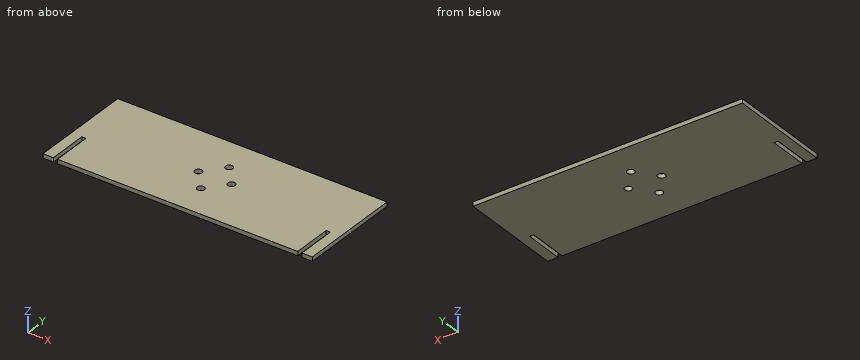
from build123d import *

# Parameters (mm, degrees)
SKETCH1_R           = 1.75
BOSS_EXTRUDE1_DEPTH = 1


with BuildPart() as part:
    # Sketch1 → Boss-Extrude1 (new, symmetric)
    with BuildSketch(Plane.XY):
        Polygon((-65, 25), (65, 25), (65, -25), (60, -25), (60, -6), (58, -6), (58, -25), (-58, -25), (-58, -6), (-60, -6), (-60, -25), (-65, -25), align=None)
        with Locations((0, 9.5)):
            Circle(SKETCH1_R, mode=Mode.SUBTRACT)
        with Locations((8, 0)):
            Circle(SKETCH1_R, mode=Mode.SUBTRACT)
        with Locations((0, -9.5)):
            Circle(SKETCH1_R, mode=Mode.SUBTRACT)
        with Locations((-8, 0)):
            Circle(SKETCH1_R, mode=Mode.SUBTRACT)
    extrude(amount=BOSS_EXTRUDE1_DEPTH, both=True)


solid = part.part
CAD build for the part. Positions are in the model's coordinates, mm. Give positions to 0.01 mm unless a question says otherwise; leave off trailing zeros. Write each loop counter-clockwise with the first axis right and the second up, starting at its lowest first coordinate (ties: lowest second). Pieces come first, ordered by that corner, then holes. Notation, with made-up numbers: (59, 17.5) -> (100, 17.5) arc R13 ccw to (100, 34.5) -> close; hole circle Ø3 at (54, 36). An arc over 180 degrees is marked (long way). Return JSON: item names as keys, results as strings.
Item 1: Band-saw the part on A-A (y = -20). List the corners of the cut face in (x, z), then the cut area to 3 significant figures.
Answer below:
{"outline": "(-65, -1) -> (-60, -1) -> (-60, 1) -> (-65, 1) -> close; (-58, -1) -> (58, -1) -> (58, 1) -> (-58, 1) -> close; (60, -1) -> (65, -1) -> (65, 1) -> (60, 1) -> close", "area": "252 mm2"}
Item 2: Band-saw the part on B-B (x = 0). List the corners of the cut face in (y, z), then the cut area to 3 significant figures.
Answer below:
{"outline": "(-25, -1) -> (-11.25, -1) -> (-11.25, 1) -> (-25, 1) -> close; (-7.75, -1) -> (7.75, -1) -> (7.75, 1) -> (-7.75, 1) -> close; (11.25, -1) -> (25, -1) -> (25, 1) -> (11.25, 1) -> close", "area": "86.0 mm2"}
Item 3: Band-saw the part on C-C (y = -9.5). List the corners of the cut face in (x, z).
Answer below:
{"outline": "(-65, -1) -> (-60, -1) -> (-60, 1) -> (-65, 1) -> close; (-58, -1) -> (-1.75, -1) -> (-1.75, 1) -> (-58, 1) -> close; (1.75, -1) -> (58, -1) -> (58, 1) -> (1.75, 1) -> close; (60, -1) -> (65, -1) -> (65, 1) -> (60, 1) -> close"}
Item 4: Drill centre lines: probe 1 along Y at (x, z) = (0, 0); probe 2 along X at (y, z) = (-21.5, -0.6); probe 3 along X at (y, z) = (-8, 0.95). Where is each one in solid material? Low to high.
Answer below:
{"probe 1": "y = -25 to -11.25, -7.75 to 7.75, 11.25 to 25", "probe 2": "x = -65 to -60, -58 to 58, 60 to 65", "probe 3": "x = -65 to -60, -58 to -0.9, 0.9 to 58, 60 to 65"}
Item 5: Drop a flat-ended pin along its axis: pin 1 (4 mm diameter, centred on x = 8, y = 0, fed in from +Z). Give the stop position or say it passes through.
Answer below:
{"pin 1": "stops at z = 1"}
Item 6: Band-saw the part on D-D (z = 0.6). List the corners of the cut face in (x, y), then the cut area to 3 significant figures.
Answer below:
{"outline": "(-65, -25) -> (-60, -25) -> (-60, -6) -> (-58, -6) -> (-58, -25) -> (58, -25) -> (58, -6) -> (60, -6) -> (60, -25) -> (65, -25) -> (65, 25) -> (-65, 25) -> close; hole circle Ø3.5 at (-8, 0); hole circle Ø3.5 at (0, -9.5); hole circle Ø3.5 at (0, 9.5); hole circle Ø3.5 at (8, 0)", "area": "6,390 mm2"}
